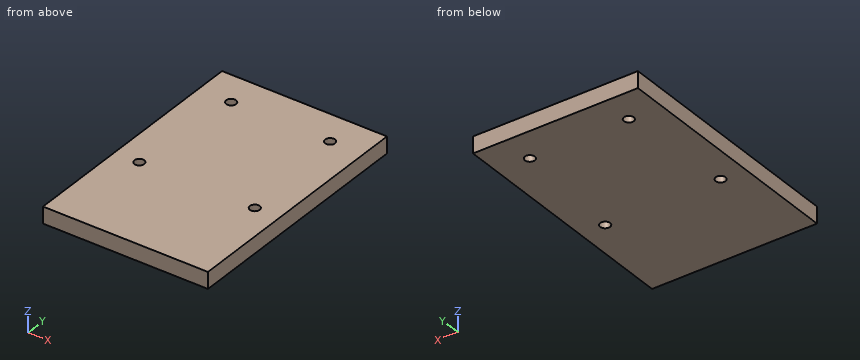
Autodesk Inventor part; units mm, degrees
ref_plane "YZ Plane" through (0, 0, 0) normal (1, 0, 0) x (0, 1, 0)
ref_plane "XZ Plane" through (0, 0, 0) normal (0, 1, 0) x (-1, 0, 0)
ref_plane "XY Plane" through (0, 0, 0) normal (0, 0, 1) x (1, 0, 0)
sketch "Sketch1" plane through (0, 0, 0) normal (0, 0, 1) x (1, 0, 0)
  line L0 (0, 0) -> (50, 0)
  line L1 (50, 0) -> (50, 75)
  line L2 (50, 75) -> (0, 75)
  line L3 (0, 75) -> (0, 0)
  line L4 (10, 65) -> (40, 65) construction
  line L5 (40, 65) -> (42.5, 30) construction
  line L6 (42.5, 30) -> (7.5, 30) construction
  line L7 (7.5, 30) -> (10, 65) construction
  line L8 (8.75, 47.5) -> (41.25, 47.5) construction
  line L9 (25, 65) -> (25, 30) construction
  circle A0 centre (10, 65) radius 1.5
  circle A1 centre (7.5, 30) radius 1.5
  circle A2 centre (42.5, 30) radius 1.5
  circle A3 centre (40, 65) radius 1.5
  point P0 (25, 75)
  dimension "d0" = 50
  dimension "d1" = 75
  dimension "d2" = 35
  dimension "d4" = 3
  dimension "d5" = 3
  dimension "d6" = 3
  dimension "d7" = 3
  dimension "d8" = 10
  dimension "d11" = 30
  dimension "d12" = 35
extrude "Extrusion1" add sketch "Sketch1" along normal blind 5
properties part number "GA006" material "ABS Plastic"
The listing builds one solid part. Answer for the finished solid, in the listing's coordinates (mm). Coordinates: 2 decimals unless noted, no trailing zeros. Order: outer loops, then holes, each group sorted by start corner. A loop starts at its lowest first (then second) coordinate and runs counter-clockwise, first axis right, second up. Notation, with made-up numbers: M -39,-24.5 L -35,-24.5 A25 ccw -35,-8.5 Z; hole C -5.75,23 d6. An arc over 180 degrees is marked long. Use CSV: the item, a comma, the result in double quotes.
Q1. Section B-B (y = 30) is taken. Determine the outline of the cut face in (x, z).
Here are the results:
outline,"M 0,0 L 6,0 L 6,5 L 0,5 Z; M 9,0 L 41,0 L 41,5 L 9,5 Z; M 44,0 L 50,0 L 50,5 L 44,5 Z"
Q2. Section A-A (x = 40) is taken. Determine the outline of the cut face in (y, z), then the cut area to 3 significant figures.
Here are the results:
outline,"M 0,0 L 63.5,0 L 63.5,5 L 0,5 Z; M 66.5,0 L 75,0 L 75,5 L 66.5,5 Z"
area,"360 mm2"
Q3. Given pin 1 Ø1.8 at (x, y) = (7.5, 30) entering from +Z, flat-ended and moving along its own axis, determine where the tip first touches the part or whether it passes through.
Here are the results:
pin 1,"through"
Q4. Straight lines are drawn through the part: L1, parallel to X at y = 65, z = 1.8; L2, parallel to Y at x = 10, z = 1.3; L3, parallel to Y at x = 42.5, z = 2.1. For each, find the intervals that lie inside material, in ascending order.
Here are the results:
L1,"0 to 8.5, 11.5 to 38.5, 41.5 to 50"
L2,"0 to 63.5, 66.5 to 75"
L3,"0 to 28.5, 31.5 to 75"
